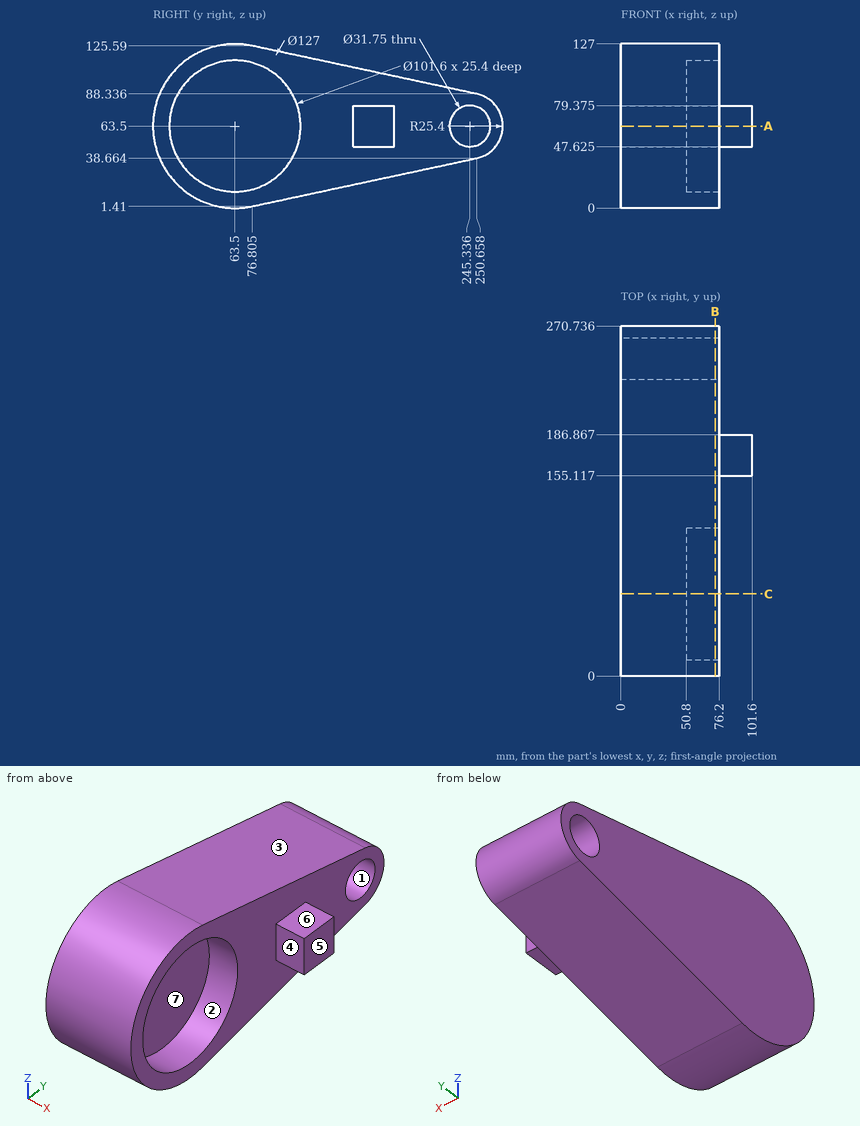
Verification items for this drawing (mm, ordinates from the low corner). A direction names the side the tool comes from. Coordinates: 2 decimals unless noted, no trailing zeros. Order: outer loops, then holes, each group sorted by start corner. A loop starts at its lowest first (then second) coordinate and runs counter-clockwise, first axis right, second up. Notation, with made-up numbers: M 19,83 L 39,83 A29 ccw 39,121 Z; hole C 24.5,20 d7. An arc over 180 degrees is marked long. Answer as a JSON object with one key per item and string values.
Q1. Cross-section at A-A on z = 63.5. Record the cut outline in (x, y), and give its area (3 significant figures).
Results are:
{"outline": "M 0,0 L 76.2,0 L 76.2,12.7 L 50.8,12.7 L 50.8,114.3 L 76.2,114.3 L 76.2,155.12 L 101.6,155.12 L 101.6,186.87 L 76.2,186.87 L 76.2,229.46 L 0,229.46 Z; M 0,261.21 L 76.2,261.21 L 76.2,270.74 L 0,270.74 Z", "area": "16,400 mm²"}
Q2. Release check for a two-part mould opening along Y. For the marked faces 1, 2, 3 and 4 record: released by +Y, released by -Y, zero draft, split by the parting line, or undercut.
Results are:
{"face 1": "undercut", "face 2": "undercut", "face 3": "released by +Y", "face 4": "released by -Y"}
Q3. Scan lines: line 1 (Y direction, x = 67, z = 63); line 2 (Z direction, x = 62, y = 63.5); line 3 (Y direction, x = 60, z = 70) (1 decimal). Record each from-to range of solid material in increasing order.
Results are:
{"line 1": "y = 0 to 12.7, 114.3 to 229.47, 261.2 to 270.73", "line 2": "z = 0 to 12.7, 114.3 to 127", "line 3": "y = 0.3 to 13.1, 113.9 to 230.9, 259.8 to 269.9"}
Q4. Cross-section at C-C on y = 63.5. Record the cut outline in (x, z).
Results are:
{"outline": "M 0,0 L 76.2,0 L 76.2,12.7 L 50.8,12.7 L 50.8,114.3 L 76.2,114.3 L 76.2,127 L 0,127 Z"}
Q5. Tool access check on the marked faces 5, 6 and 7. Record the directions out of +Z, -Z, +X, -X, +Y, -Y that give a thin tool (end or side, any length) a straight path to the whole face; none if there is none.
Results are:
{"face 5": "+Z, -Z, +X, +Y, -Y", "face 6": "+Z, +X, +Y, -Y", "face 7": "+X"}
Q6. Depth check by flat-ended pin: pin 1 Ø12 at (x, z) = (49, 87) entering from -Y; pin 2 Ø8 at (x, y) = (34, 211) entering from +Z; pin 3 Ø3 at (x, y) = (41.5, 206.5) entering from -Z. Enter the tip coordinate at first touch or a pass-through.
Results are:
{"pin 1": "stops at y = 2.46", "pin 2": "stops at z = 97.69", "pin 3": "stops at z = 28.88"}
Q7. Cross-section at B-B on x = 73. Give the number of separate pieces and of enclosed holes in the cut face, and give its area (3 significant figures).
Results are:
{"separate pieces": "1", "enclosed holes": "2", "area": "15,000 mm²"}
